Read the model definition and answer for the solid it produces. Units are mm, in the model's axes. A direction names the side the tool comes from. Coordinates: 2 decimals unless noted, no trailing zeros. Loops run counter-clockwise (first coordinate to the right, second up) from the corner with the lowest first, then second, coordinate; pieces in that order, holes last. Notation, with made-up numbers: (-20, 40) -> (-15, 40) arc R12 ccw to (-15, 60) -> close; hole circle Ø1 at (17, 9.25). An arc over 180 degrees is marked (long way). Answer as a JSON object with one key per item and string values. Group by question number.
1) Section C-C, the plane z = 3.1 is taken. Give the vertices of the cut face in (x, y), plus the area to 3 significant figures.
2) Section A-A, the plane x = 14.5 is taken. Give the vertices of the cut face in (y, z).
3) Section D-D, the plane y = 23.5 is taken. Give the vertices of the cut face in (x, z), plus the area to 3 significant figures.
4) Which of the six approach directions +Z, -Z, +X, -X, +Y, -Y give full straight-line access (tool end or side, diameter ignored) to faces 5 (the face through (99.753, 18.833, 2.521)), 6 (the face through (54, 17, 0)), 7 (the face through (19, 26.19, 2))?
5) Consider probe 1 along Y at (x, z) = (103, 0.7); probe 2 along Y at (x, z) = (103, 2.35); probe 3 along X at (y, z) = (29, 2.8). Determine where each line is inside the solid, lowest interval first. Write a range as [from, to].
6) Section B-B, the plane y = 18.69 is taken. Give the vertices of the cut face in (x, z), plus the area to 3 significant figures.
7) Flat-ended cylindrical pins translate along their axes: P1, Ø1, axis at y = 15, z = 1, coming from the -X side; P2, Ø5.5, axis at x = 103, y = 18.69, coming from the -Z side; P3, Ø0.6, axis at y = 29, z = 1, coming from the +X side; P4, Ø2, axis at y = 29.5, z = 2.5, coming from the -X side. Find the tip coordinate at first contact, or state that the pin passes through.
8) Determine the mould class of faces 1 (the face through (4.605, 20.887, 2.521)), 2 (the face through (108.859, 16.987, 2.797)), 3 (the face through (1.203, 16.987, 2.859)), 4 (the face through (8, 17, 1)) for opening direction X: released by +X, released by -X, zero draft, split by the parting line, or undercut.
from build123d import *

# Parameters (mm, degrees)
ESQUISSE1_W             = 110
ESQUISSE1_H             = 34.19
BOSS_EXTRU_1_DEPTH      = 4
BOSS_EXTRU_2_DEPTH      = 110
ESQUISSE3_R             = 1.75
ENL_V_MAT_EXTRU_1_DEPTH = 4
ESQUISSE4_R             = 3.25
ENL_V_MAT_EXTRU_2_DEPTH = 3
ENL_V_MAT_EXTRU_3_DEPTH = 4
CONG_1_R                = 4


with BuildPart() as part:
    # Esquisse1 → Boss.-Extru.1 (new body)
    with BuildSketch(Plane.XY):
        with Locations((55, 17.095)):
            Rectangle(ESQUISSE1_W, ESQUISSE1_H)
    extrude(amount=BOSS_EXTRU_1_DEPTH)

    # Esquisse2 → Boss.-Extru.2 (add)
    with BuildSketch(Plane(origin=(110, 0, 0), x_dir=(0, 0, -1), z_dir=(1, 0, 0))):
        Polygon((0, 0), (-4, 0), (-4, -0.705307923), align=None)
    extrude(amount=-BOSS_EXTRU_2_DEPTH)

    # Esquisse3 → Enlèv. mat.-Extru.1 (cut)
    with BuildSketch(Plane.XY.offset(4)):
        with Locations((7, 18.69)):
            Circle(ESQUISSE3_R)
        with Locations((103, 18.69)):
            Circle(ESQUISSE3_R)
    extrude(amount=-ENL_V_MAT_EXTRU_1_DEPTH, mode=Mode.SUBTRACT)

    # Esquisse4 → Enlèv. mat.-Extru.2 (cut)
    with BuildSketch(Plane.XY.offset(4)):
        with Locations((7, 18.69)):
            Circle(ESQUISSE4_R)
        with Locations((103, 18.69)):
            Circle(ESQUISSE4_R)
    extrude(amount=-ENL_V_MAT_EXTRU_2_DEPTH, mode=Mode.SUBTRACT)

    # Esquisse5 → Enlèv. mat.-Extru.3 (cut)
    with BuildSketch(Plane.XY.offset(4)):
        with BuildLine():
            Line((12.5, 32.19), (24.5, 32.19))
            ThreePointArc((24.5, 32.19), (25.914213562, 31.604213562), (26.5, 30.19))
            Line((26.5, 30.19), (26.5, 28.19))
            ThreePointArc((26.5, 28.19), (25.914213562, 26.775786438), (24.5, 26.19))
            Line((24.5, 26.19), (12.5, 26.19))
            ThreePointArc((12.5, 26.19), (11.085786438, 26.775786438), (10.5, 28.19))
            Line((10.5, 28.19), (10.5, 30.19))
            ThreePointArc((10.5, 30.19), (11.085786438, 31.604213562), (12.5, 32.19))
        make_face()
    extrude(amount=-ENL_V_MAT_EXTRU_3_DEPTH, mode=Mode.SUBTRACT)

    # Congé1
    # the kernel refuses this fillet: 4 mm, written as the material it takes off along each edge
    with BuildSketch(Plane(origin=(0, 44.19, 4), x_dir=(1, 0, 0), z_dir=(0, -1, 0)), Plane(origin=(110, 44.19, 4), x_dir=(0, 0, -1), z_dir=(0, -1, 0))) as cong_1_piece_1:
        with BuildLine():
            CenterArc((CONG_1_R, -CONG_1_R), CONG_1_R, 90, 90)
            Line((0, -CONG_1_R), (0, 0))
            Line((0, 0), (CONG_1_R, 0))
        make_face()
    extrude(amount=54.895307923, mode=Mode.SUBTRACT)


solid = part.part
Determined:
{
 "1": {"outline": "(1.47, -0.55) -> (108.53, -0.55) -> (108.53, 34.19) -> (1.47, 34.19) -> close; hole circle Ø6.5 at (7, 18.69); hole (10.5, 28.19) arc R2 ccw to (12.5, 26.19) -> (24.5, 26.19) arc R2 ccw to (26.5, 28.19) -> (26.5, 30.19) arc R2 ccw to (24.5, 32.19) -> (12.5, 32.19) arc R2 ccw to (10.5, 30.19) -> close; hole circle Ø6.5 at (103, 18.69)", "area": "3,560 mm²"},
 "2": {"outline": "(-0.71, 4) -> (0, 0) -> (26.19, 0) -> (26.19, 4) -> close; (32.19, 0) -> (34.19, 0) -> (34.19, 4) -> (32.19, 4) -> close"},
 "3": {"outline": "(0, 0) -> (110, 0) arc R4 ccw to (106, 4) -> (4, 4) arc R4 ccw to start", "area": "433 mm²"},
 "4": {"face 5": "+Z", "face 6": "-Z, +X, -X, +Y, -Y", "face 7": "+Z, -Z"},
 "5": {"probe 1": "[-0.12, 16.94], [20.44, 34.19]", "probe 2": "[-0.41, 15.44], [21.94, 34.19]", "probe 3": "[1.14, 10.5], [26.5, 108.86]"},
 "6": {"outline": "(0, 0) -> (5.25, 0) -> (5.25, 1) -> (3.75, 1) -> (3.75, 3.99) arc R4 ccw to start; (8.75, 0) -> (101.25, 0) -> (101.25, 1) -> (99.75, 1) -> (99.75, 4) -> (10.25, 4) -> (10.25, 1) -> (8.75, 1) -> close; (104.75, 0) -> (110, 0) arc R4 ccw to (106.25, 3.99) -> (106.25, 1) -> (104.75, 1) -> close", "area": "387 mm²"},
 "7": {"P1": "x = 0.03", "P2": "z = 0", "P3": "x = 109.94", "P4": "x = 0.29"},
 "8": {"face 1": "undercut", "face 2": "released by +X", "face 3": "released by -X", "face 4": "undercut"}
}
